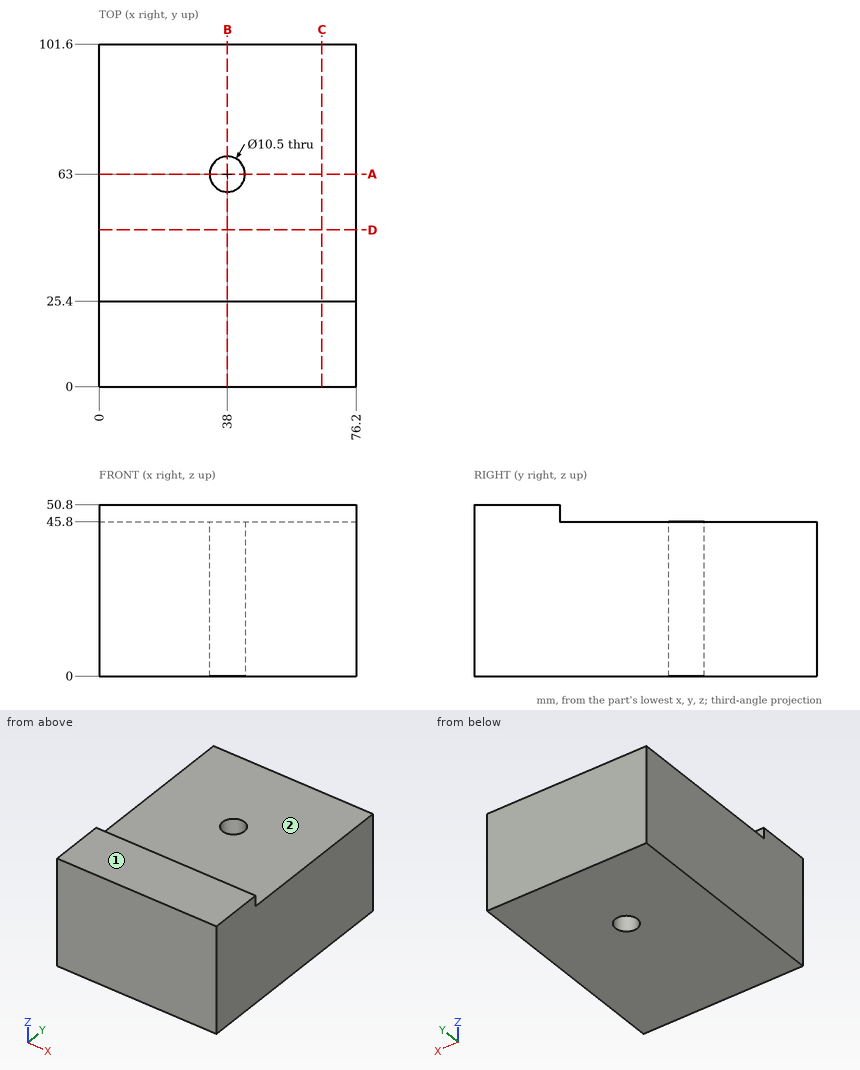
Geometry: see drawing. Coordinates: mm, zero at the bounding-box minimum. A direction names the side the tool comes from. Coordinates: 2 decimals unless noted, no trailing zeros. Loops run counter-clockwise (first coordinate to the right, second up) from the corner with the lowest first, then second, coordinate; pieces in that order, holes last. Notation, with made-up numbers: (6.5, -17.5) -> (49.5, -17.5) arc R28 ccw to (49.5, 1.5) -> close; hole circle Ø3 at (-22, 11). An arc over 180 degrees is marked (long way). Write item = value, one per line. Start each with the question number.
Item 1: Cut plane D-D, the plane y = 46.5. Return loops of the section in (x, z).
Item 2: Cut plane B-B, the plane x = 38. Return loops of the section in (y, z).
Item 3: Reachability of the marked faces 1 and 2 from +Z, -Z, +X, -X, +Y, -Y: full face, straight path, thin tool, end or side. Return the list, or none.
Item 4: First-contact query: P1, Ø2.5, axis at x = 49, z = 49, coming from the +Y side; P2, Ø23, axis at x = 33.5, y = 53, coming from the +Z side. Flat tips, straight axial feed; report the tip coordinate or a pass-through.
Item 5: Material intervals for line 1 (Y direction, x = 38.5, z = 13); line 2 (Z direction, x = 34, y = 36); line 3 (Y direction, x = 34, z = 25), sorted ascending.
Item 6: Cut plane A-A, the plane y = 63. Return loops of the section in (x, z).
Item 7: Cut plane C-C, the plane x = 66. Return loops of the section in (y, z).
Ans:
q1.outline = (0, 0) -> (76.2, 0) -> (76.2, 45.8) -> (0, 45.8) -> close
q2.outline = (0, 0) -> (57.75, 0) -> (57.75, 45.8) -> (25.4, 45.8) -> (25.4, 50.8) -> (0, 50.8) -> close; (68.25, 0) -> (101.6, 0) -> (101.6, 45.8) -> (68.25, 45.8) -> close
q3.face_1 = +Z, +X, -X, +Y, -Y
q3.face_2 = +Z, +X, -X, +Y
q4.P1 = 25.4
q4.P2 = 45.8
q5.line_1 = 0 to 57.77, 68.23 to 101.6
q5.line_2 = 0 to 45.8
q5.line_3 = 0 to 59.6, 66.4 to 101.6
q6.outline = (0, 0) -> (32.75, 0) -> (32.75, 45.8) -> (0, 45.8) -> close; (43.25, 0) -> (76.2, 0) -> (76.2, 45.8) -> (43.25, 45.8) -> close
q7.outline = (0, 0) -> (101.6, 0) -> (101.6, 45.8) -> (25.4, 45.8) -> (25.4, 50.8) -> (0, 50.8) -> close
